Autodesk Inventor part; units mm, degrees
ref_plane "YZ Plane" through (0, 0, 0) normal (1, 0, 0) x (0, 1, 0)
ref_plane "XZ Plane" through (0, 0, 0) normal (0, 1, 0) x (-1, 0, 0)
ref_plane "XY Plane" through (0, 0, 0) normal (0, 0, 1) x (1, 0, 0)
sketch "Эскиз2" plane through (0, 0, 0) normal (0, 0, 1) x (1, 0, 0)
  line L0 (0, 0) -> (12, 0)
  line L1 (12, 0) -> (12, 10)
  line L2 (12, 10) -> (0, 10)
  line L3 (0, 10) -> (0, 0)
  line L4 (-15.2128, 15.4518) -> (-15.9082, 15.4518)
  line L5 (-15.9082, 15.4518) -> (-15.9082, 15.4083)
  line L6 (-15.9082, 15.4083) -> (-15.2128, 15.4083)
  line L7 (-15.2128, 15.4083) -> (-15.2128, 15.4518)
  dimension "d0" = 12
  dimension "d1" = 10
extrude "Выдавливание1" add sketch "Эскиз2" along normal blind 1 contours L3 L2 L1 L0
sketch "Эскиз3" plane through (0, 0, 1) normal (0, 0, 1) x (1, 0, 0)
  line L0 (0, 10) -> (0, 0)
  line L1 (0, 5) -> (12, 5)
  line L2 (12, 0) -> (12, 10)
  circle A0 centre (6, 5) radius 2
  dimension "d4" = 4
extrude "Выдавливание2" add sketch "Эскиз3" along normal blind 0.7
sketch "Эскиз5" plane through (0, 0, 0) normal (0, 0, -1) x (-1, 0, 0)
  line L0 (-12, 10) -> (0, 10)
  line L1 (0, 10) -> (0, 0)
  line L2 (-12, 10) -> (0, 10)
  line L3 (0, 10) -> (0, 0)
  line L4 (0, 0) -> (-12, 0)
  line L5 (-12, 0) -> (-12, 10)
  line L6 (-12, 10) -> (-11, 10)
  line L7 (-11, 10) -> (-11, 9)
  line L8 (-11, 9) -> (-1, 9)
  line L9 (-1, 9) -> (-1, 1)
  line L10 (-1, 1) -> (-11, 1)
  line L11 (-11, 1) -> (-11, 9)
  dimension "d22" = 1
  dimension "d23" = 1
  dimension "d24" = 10
  dimension "d25" = 8
  dimension "d26" = 12
  dimension "d27" = 10
extrude "Выдавливание4" add sketch "Эскиз5" along normal blind 8 contours L8 L9 L10 L11
sketch "Эскиз6" plane through (0, 0, -8) normal (0, 0, -1) x (-1, 0, 0)
  line L0 (-12, 10) -> (0, 10)
  line L1 (0, 10) -> (0, 0)
  line L2 (-12, 10) -> (0, 10)
  line L3 (0, 10) -> (0, 0)
  line L4 (0, 0) -> (-12, 0)
  line L5 (-12, 0) -> (-12, 10)
extrude "Выдавливание5" add sketch "Эскиз6" along normal blind 15
sketch "Эскиз11" plane through (6, 5, 1.7) normal (0, 0, 1) x (1, 0, 0)
  circle A0 centre (0, 0) radius 1.5
  point P0 (-6, -5)
  dimension "d32" = 3
extrude "Выдавливание9" cut sketch "Эскиз11" against normal blind 1
sketch "Эскиз8" plane through (0, 0, -23) normal (0, 0, -1) x (-1, 0, 0)
  circle A0 centre (-6, 5) radius 2
  circle A1 centre (-6, 5) radius 2.5
  point P0 (0, 0)
  dimension "d15" = 5
extrude "Выдавливание6" add sketch "Эскиз8" along normal blind 0.5 contours A0
equation "\"d22\" = -0.5 * d24 + 0.5 * d26"
equation "\"d23\" = -0.5 * d25 + 0.5 * d27"
properties part number "Micro Gearmotors"
For this review, take the finished solid that the model builds, in its own axes (mm). A direction names the side the tool comes from. Give positions to 0.01 mm unless a question says otherwise; leave off trailing zeros. Loops run counter-clockwise (first coordinate to the right, second up) from the corner with the lowest first, then second, coordinate; pieces in that order, holes last.
Item 1: Tool access review of faces 1 (the flat face through (11, 5, -4)), 2 (the flat face through (6.1, 7.3, -23)), 3 (the flat face through (1, 5, -4)), 4 (the flat face through (5.9, 7.3, 1)), 5 (the flat face through (6, 9, -4)): name each direction out of +Z, -Z, +X, -X, +Y, -Y from which nothing blocks a thin tool from reaching the whole face with its end or side.
Item 2: For line 1 along Z through (x, y) = (1.5, 0.5); line 2 along Y through (x, z) = (6, 1.2); line 3 along Z through (x, y) = (9, 1.25), list the stretches that pass through material, from the lowest coordinate up.
Item 3: Take a section at B-B, the plane y = 1.5. State the section outline as (x, z) points.
Item 4: Insertion check: pin 1 (4 mm diameter, centred on y = 7, z = -5.5, fed in from +X); pin 2 (1.5 mm diameter, centred on x = 6.5, y = 4.5, fed in from +Z); pin 3 (1 mm diameter, centred on x = 3.5, y = 8.5, fed in from +Z). Each pin has a flat end and moves straight along its axis. Give the tip position at first contact, or say it passes through.
Item 5: Take a section at C-C, the plane z = -0.25. State the section outline as (x, y) points, and give its area (3 significant figures).
Item 6: Take a section at A-A, the plane x = 6. State the section outline as (y, z) points.
Item 7: Draft analysis for pull direction X (two halves, no side actions). For faces 6 (the cylindrical face through (4.8, 4.1, 1.2)), 7 (the cylindrical face through (7.6, 6.2, -23.2)), 8 (the flat face through (6, 5, 0.7)), 9 (the flat face through (0, 5, -15)), state which applies: +X half, -X half, draft (parallel to the pull), parting line (faces both ways), or undercut.
Item 8: Take a section at D-D, the plane x = 10. State the section outline as (y, z) points, and give its area (3 significant figures).
Calculated:
1. face 1: +X, +Y, -Y
1. face 2: -Z
1. face 3: -X, +Y, -Y
1. face 4: +Z
1. face 5: +X, -X, +Y
2. line 1: z = -23 to -8, 0 to 1
2. line 2: y = 3 to 3.5, 6.5 to 7
2. line 3: z = -23 to 1
3. outline: (0, -23) - (12, -23) - (12, -8) - (11, -8) - (11, 0) - (12, 0) - (12, 1) - (0, 1) - (0, 0) - (1, 0) - (1, -8) - (0, -8) - close
4. pin 1: stops at x = 11
4. pin 2: stops at z = 0.7
4. pin 3: stops at z = 1
5. outline: (1, 1) - (11, 1) - (11, 9) - (1, 9) - close
5. area: 80.0 mm2
6. outline: (0, -23) - (3, -23) - (3, -23.5) - (7, -23.5) - (7, -23) - (10, -23) - (10, -8) - (9, -8) - (9, 0) - (10, 0) - (10, 1) - (7, 1) - (7, 1.7) - (6.5, 1.7) - (6.5, 0.7) - (3.5, 0.7) - (3.5, 1.7) - (3, 1.7) - (3, 1) - (0, 1) - (0, 0) - (1, 0) - (1, -8) - (0, -8) - close
7. face 6: undercut
7. face 7: parting line
7. face 8: undercut
7. face 9: -X half
8. outline: (0, -23) - (10, -23) - (10, -8) - (9, -8) - (9, 0) - (10, 0) - (10, 1) - (0, 1) - (0, 0) - (1, 0) - (1, -8) - (0, -8) - close
8. area: 224 mm2
